from build123d import *

# Parameters (mm, degrees)
SKETCH1_W           = 25.4
SKETCH1_H           = 25.4
BOSS_EXTRUDE1_DEPTH = 3.81
SKETCH2_W           = 7.62
SKETCH2_H           = 25.4
BOSS_EXTRUDE2_DEPTH = 2.54


with BuildPart() as part:
    # Sketch1 → Boss-Extrude1 (new body)
    with BuildSketch(Plane(origin=(0, 0, 0), x_dir=(0, 0, -1), z_dir=(1, 0, 0))):
        with Locations((-12.7, 12.7)):
            Rectangle(SKETCH1_W, SKETCH1_H)
    boss_extrude1 = extrude(amount=BOSS_EXTRUDE1_DEPTH)

    # Sketch2 → Boss-Extrude2 (add)
    with BuildSketch(Plane.XY):
        with Locations((-3.81, 12.7)):
            Rectangle(SKETCH2_W, SKETCH2_H)
    boss_extrude2 = extrude(amount=BOSS_EXTRUDE2_DEPTH)

    # Mirror2: Boss-Extrude1, Boss-Extrude2 across plane
    add(boss_extrude1.mirror(Plane(origin=(3.81, 0, 0), x_dir=(0, 0, 1), z_dir=(1, 0, 0))))
    add(boss_extrude2.mirror(Plane(origin=(3.81, 0, 0), x_dir=(0, 0, 1), z_dir=(1, 0, 0))))


solid = part.part
Could you check a few things on this model? Use its own coordinates, in mm. A direction names the side the tool comes from. Give positions to 0.01 mm unless a question says otherwise; leave off trailing zeros. Order: outer loops, then holes, each group sorted by start corner. A loop starts at its lowest first (then second) coordinate and runs counter-clockwise, first axis right, second up. Notation, with made-up numbers: (3, 84) -> (20, 84) arc R15 cw to (20, 103) -> close; hole circle Ø6 at (42, 24). An arc over 180 degrees is marked (long way). Return JSON: item names as keys, results as strings.
1. Imagine slicing it at B-B on x = 13. List the corners of the cut face in (y, z) for me.
Answer list:
{"outline": "(0, 0) -> (25.4, 0) -> (25.4, 2.54) -> (0, 2.54) -> close"}
2. Imagine slicing it at C-C on z = 10.75. List the corners of the cut face in (x, y) for me.
Answer list:
{"outline": "(0, 0) -> (7.62, 0) -> (7.62, 25.4) -> (0, 25.4) -> close"}
3. Imagine slicing it at A-A on y = 15.25. List the corners of the cut face in (x, z) for me, then the cut area to 3 significant figures.
Answer list:
{"outline": "(-7.62, 0) -> (15.24, 0) -> (15.24, 2.54) -> (7.62, 2.54) -> (7.62, 25.4) -> (0, 25.4) -> (0, 2.54) -> (-7.62, 2.54) -> close", "area": "232 mm2"}
4. I need wall thicknesses on line 1 (X direction, y = 14.5, z = 12.5); line 2 (Z direction, x = -5.75, y = 24.75). Which ranges of each line are inside material? Lowest first, please. Write a range as from..to.
Answer list:
{"line 1": "x = 0..7.62", "line 2": "z = 0..2.54"}
5. On a 3-axis mill with a long thin cutter (end or side, diameter ignored), from which of +Z, -Z, +X, -X, +Y, -Y can I reach the whole of each face in a straight line? I mean faces 1 (the flat face through (4, 13, 0)), 2 (the flat face through (7.62, 13, 14)), 3 (the flat face through (-4, 13, 2.54)). Say none if no direction works.
Answer list:
{"face 1": "-Z, +X, -X, +Y, -Y", "face 2": "+Z, +X, +Y, -Y", "face 3": "+Z, -X, +Y, -Y"}
6. For pin 1 Ø3 at (y, z) = (9, 7) entering from -X; pin 2 Ø2 at (x, y) = (-1, 13.5) entering from -Z; pin 3 Ø1 at (x, y) = (12, 18.5) entering from +Z, each with a flat end and sliding along its axis, tell me the tip position at first contact or that it passes through.
Answer list:
{"pin 1": "stops at x = 0", "pin 2": "stops at z = 0", "pin 3": "stops at z = 2.54"}
